Part model, mm, in its own coordinate system. A direction names the side the tool comes from. Coordinates: 2 decimals unless noted, no trailing zeros. Write each loop counter-clockwise with the first axis right and the second up, starting at its lowest first coordinate (ties: lowest second). Pieces come first, ordered by that corner, then holes. Notation, with made-up numbers: M 1.5,66.5 L 26.5,66.5 A13 ccw 26.5,87.5 Z; hole C 54.25,3.5 d10. An arc over 180 degrees is marked long. Use a Markdown table: item, result. Add a question column.
Q1. Slice it at D-D on z = 15. Write the cut outline in (x, y), then the cut area to 3 significant figures.
Q2. Wall check: L1, parallel to X at y = 1.65, z = 6; L2, parallel to X at y = 2.6, z = 0; L3, parallel to X at y = 13.75, z = -7. Give the ranges that are in metal, low to high. Write a range as from..to.
Q3. Tool access for faces 1 (the flat face through (35, 9, 0)), 2 (the flat face through (-31, 9, 0)), 3 (the flat face through (-33, 9, 30)): list every direction of +Z, -Z, +X, -X, +Y, -Y with a clear straight run to the whole face (end or side of a thin tool).
Q4. Slice it at A-A on x = 0. Write the cut outline in (y, z).
Q5. Mould opens along Y. For faces 4 (the cylindrical face through (0.466, 1.972, -43.272)), 5 (the flat face through (-33, 14, 0)), 6 (the cylindrical face through (32.972, 11.082, 6.727)) say: released by +Y, released by -Y, zero draft, split by the parting line, or undercut.
Q6. Slice it at B-B on z = -12. Write the cut outline in (x, y), then the cut area to 3 significant figures.
Q7. Slice it at C-C on x = 44.75. Write the cut outline in (y, z).
Q8. Pin check, flat tips, straight feed: pin 1 Ø5 at (x, z) = (0, -44.75) entering from +Y; pin 2 Ø5 at (y, z) = (9, 7) entering from -X; pin 3 Ø3.5 at (y, z) = (9, 21) entering from +X; pin 4 Ø5 at (y, z) = (7, -1) entering from +X. Stop position of each tip, or through.
from build123d import *

# Parameters (mm, degrees)
SKETCH_1_R             = 53.491930893
SKETCH_1_R_2           = 1.55
SKETCH_1_R_3           = 1.6
EXTRUDE_563_DEPTH      = 4
SKETCH_2_W             = 4
SKETCH_2_H             = 60
EXTRUDE_829_DEPTH      = 10
SKETCH_3_R             = 2.1
CUT_EXTRUDE_1129_DEPTH = 105.346578783


with BuildPart() as part:
    # 草图1 → Extrude 563 (new body)
    with BuildSketch(Plane(origin=(0, 0, 0), x_dir=(1, 0, 0), z_dir=(0, 1, 0))):
        with Locations(Location((0, 0, 0), (0, 0, 270))):
            Circle(SKETCH_1_R)
        with Locations(Location((0, 44.75, 0), (0, 0, 270))):
            Circle(SKETCH_1_R_2, mode=Mode.SUBTRACT)
        with Locations(Location((-44.75, 0, 0), (0, 0, 270))):
            Circle(SKETCH_1_R_2, mode=Mode.SUBTRACT)
        with Locations(Location((44.75, 0, 0), (0, 0, 90))):
            Circle(SKETCH_1_R_2, mode=Mode.SUBTRACT)
        with Locations(Location((0, -44.75, 0), (0, 0, 90))):
            Circle(SKETCH_1_R_2, mode=Mode.SUBTRACT)
        with Locations(Location((0, 12, 0), (0, 0, 270))):
            Circle(SKETCH_1_R_3, mode=Mode.SUBTRACT)
        with Locations(Location((10.392304845, -6, 0), (0, 0, 270))):
            Circle(SKETCH_1_R_3, mode=Mode.SUBTRACT)
        with Locations(Location((-10.392304845, -6, 0), (0, 0, 270))):
            Circle(SKETCH_1_R_3, mode=Mode.SUBTRACT)
    extrude(amount=EXTRUDE_563_DEPTH)

    # 草图2 → Extrude 829 (add)
    with BuildSketch(Plane(origin=(0, 4, 0), x_dir=(1, 0, 0), z_dir=(0, 1, 0))):
        with Locations((33, 0)):
            Rectangle(SKETCH_2_W, SKETCH_2_H)
        with Locations((-33, 0)):
            Rectangle(SKETCH_2_W, SKETCH_2_H)
    extrude(amount=EXTRUDE_829_DEPTH)

    # 草图3 → Cut-Extrude 1129 (cut, through all)
    with BuildSketch(Plane.ZY.offset(35)):
        with Locations((7, 9)):
            Circle(SKETCH_3_R)
        with Locations((-7, 9)):
            Circle(SKETCH_3_R)
        with Locations((-21, 9)):
            Circle(SKETCH_3_R)
        with Locations((21, 9)):
            Circle(SKETCH_3_R)
    extrude(amount=-CUT_EXTRUDE_1129_DEPTH, mode=Mode.SUBTRACT)


solid = part.part
Recorded:
| question | item | result |
|---|---|---|
| 1 | outline | M -51.35,0 L 51.35,0 L 51.35,4 L 35,4 L 35,14 L 31,14 L 31,4 L -31,4 L -31,14 L -35,14 L -35,4 L -51.35,4 Z |
| 1 | area | 491 mm² |
| 2 | L1 | -53.15..-11.99, -8.79..8.79, 11.99..53.15 |
| 2 | L2 | -53.49..-46.3, -43.2..43.2, 46.3..53.49 |
| 2 | L3 | -35..-31, 31..35 |
| 3 | face 1 | +Z, -Z, +X, +Y |
| 3 | face 2 | +Z, -Z, +Y |
| 3 | face 3 | +Z, +X, -X, +Y |
| 4 | outline | M 0,-53.49 L 4,-53.49 L 4,-46.3 L 0,-46.3 Z; M 0,-43.2 L 4,-43.2 L 4,-13.6 L 0,-13.6 Z; M 0,-10.4 L 4,-10.4 L 4,43.2 L 0,43.2 Z; M 0,46.3 L 4,46.3 L 4,53.49 L 0,53.49 Z |
| 5 | face 4 | zero draft |
| 5 | face 5 | released by +Y |
| 5 | face 6 | undercut |
| 6 | outline | M -52.13,0 L -1.6,0 L -1.6,4 L -31,4 L -31,14 L -35,14 L -35,4 L -52.13,4 Z; M 1.6,0 L 52.13,0 L 52.13,4 L 35,4 L 35,14 L 31,14 L 31,4 L 1.6,4 Z |
| 6 | area | 484 mm² |
| 7 | outline | M 0,-29.31 L 4,-29.31 L 4,-1.55 L 0,-1.55 Z; M 0,1.55 L 4,1.55 L 4,29.31 L 0,29.31 Z |
| 8 | pin 1 | y = 4 |
| 8 | pin 2 | x = -35 |
| 8 | pin 3 | through |
| 8 | pin 4 | x = 35 |
